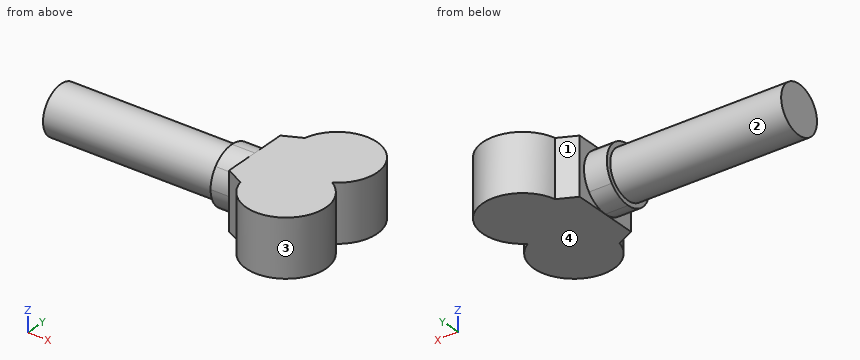
from build123d import *

# Parameters (mm, degrees)
F1_DEPTH = 2.5
F3_DEPTH = 2
F4_R     = 2.1
F5_DEPTH = 15


with BuildPart() as f1:
    # F0 (on Top) → F1 (new body, symmetric)
    with BuildSketch(Plane.XY):
        with BuildLine():
            ThreePointArc((8.1972243623, 3), (10, 2.5), (11.8027756377, 3))
            ThreePointArc((11.8027756377, 3), (10, 3.5), (8.1972243623, 3))
        make_face()
        with BuildLine():
            ThreePointArc((8.1972243623, 3), (6.7824000154, 4.6226654949), (6.584950352, 6.7664436716))
            Line((6.584950352, 6.7664436716), (5, 6))
            Line((5, 6), (5, 3))
            Line((5, 3), (5, 0))
            Line((5, 0), (6.5932639339, -0.8025891701))
            ThreePointArc((6.5932639339, -0.8025891701), (6.7751474224, 1.3602668315), (8.1972243623, 3))
        make_face()
        with BuildLine():
            ThreePointArc((11.8027756377, 3), (13.0462858313, 4.2765898242), (13.5, 6))
            ThreePointArc((13.5, 6), (10.385568562, 9.4786975844), (6.584950352, 6.7664436716))
            ThreePointArc((6.584950352, 6.7664436716), (6.7824000154, 4.6226654949), (8.1972243623, 3))
            ThreePointArc((8.1972243623, 3), (10, 3.5), (11.8027756377, 3))
        make_face()
        with BuildLine():
            ThreePointArc((13.5, 0), (13.0462858313, 1.7234101758), (11.8027756377, 3))
            ThreePointArc((11.8027756377, 3), (10, 2.5), (8.1972243623, 3))
            ThreePointArc((8.1972243623, 3), (6.7751474224, 1.3602668315), (6.5932639339, -0.8025891701))
            ThreePointArc((6.5932639339, -0.8025891701), (10.4039949063, -3.4766058327), (13.5, 0))
        make_face()
    extrude(amount=F1_DEPTH, both=True)

    # F2 (on face) → F3 (join)
    with BuildSketch(Plane(origin=(5, 0, 0), x_dir=(0, -1, 0), z_dir=(-1, 0, 0))):
        with BuildLine():
            ThreePointArc((-0.5, 0), (-0.6493210558, 0.8510631594), (-1.079446801, 1.6004609992))
            Line((-1.079446801, 1.6004609992), (-3, 0))
            Line((-3, 0), (-1.079446801, -1.6004609992))
            ThreePointArc((-1.079446801, -1.6004609992), (-0.6493210558, -0.8510631594), (-0.5, 0))
        make_face()
        with BuildLine():
            Line((-3, 0), (-1.079446801, 1.6004609992))
            ThreePointArc((-1.079446801, 1.6004609992), (-1.9396115094, 2.2639735531), (-3, 2.5))
            ThreePointArc((-3, 2.5), (-4.0603884906, 2.2639735531), (-4.920553199, 1.6004609992))
            Line((-4.920553199, 1.6004609992), (-3, 0))
        make_face()
        with BuildLine():
            Line((-1.079446801, -1.6004609992), (-3, 0))
            Line((-3, 0), (-4.920553199, -1.6004609992))
            ThreePointArc((-4.920553199, -1.6004609992), (-4.0603884906, -2.2639735531), (-3, -2.5))
            ThreePointArc((-3, -2.5), (-1.9396115094, -2.2639735531), (-1.079446801, -1.6004609992))
        make_face()
        with BuildLine():
            Line((-4.920553199, -1.6004609992), (-3, 0))
            Line((-3, 0), (-4.920553199, 1.6004609992))
            ThreePointArc((-4.920553199, 1.6004609992), (-5.5, 0), (-4.920553199, -1.6004609992))
        make_face()
    extrude(amount=F3_DEPTH)

    # F4 (on face) → F5 (join)
    with BuildSketch(Plane(origin=(3, 0, 0), x_dir=(0, -1, 0), z_dir=(-1, 0, 0))):
        with Locations((-3, 0)):
            Circle(F4_R)
    extrude(amount=F5_DEPTH)


solid = f1.part
For this review, take the finished solid that the model builds, in its own axes (mm). Face numbers are marked on the shaded views. Round coordinates to 2 decimals unless told otherwise and drop trailing zeros. Write each loop counter-clockwise with the first axis right and the second up, starting at its lowest first coordinate (ties: lowest second). Pieces come first, ordered by that corner, then holes. Notation, with made-up numbers: M 61.5,-37 L 74.5,-37 A18 ccw 74.5,-15 Z; hole C 54.25,-36 d1. An arc over 180 degrees is marked long. Write item = value, one per line. Start each with the question number.
(1) We need section B-B (z = 1.35). Give the boundary of the cut face in (x, y), then the cut area to 3 significant figures.
(2) The part is to be moulded in two halves that separate along Y. For the marked faces 1, 2, 3 and 4, say which applies: +Y half, -Y half, draft (parallel to the pull), parting line (faces both ways), or undercut.
(3) We need section C-C (y = 1.5). Give the boundary of the cut face in (x, z), then the cut area to 3 significant figures.
(4) Clearance check with flat-ended pins moving along their axes: pin 1 Ø3 at (x, y) = (-5.5, 6) entering from +Z; pin 2 Ø2 at (x, z) = (-3, -1) entering from +Y; pin 3 Ø3 at (x, y) = (-1, 2) entering from -Z. State where each tip first meets the part, or that it passes through.
(5) For line 1 along X through (y, z) = (0.5, 0.9); line 2 along Z through (x, y) = (-4.5, 1.25); line 3 along Y through (x, z) = (7.25, -1.55), list the stretches that pass through material, from the lowest coordinate up.
(6) We need section A-A (x = 4.25). Give the boundary of the cut face in (y, z), then the cut area to 3 significant figures.
(7) We need section D-D (x = -9.5). Give the boundary of the cut face in (y, z), then the cut area to 3 significant figures.
Results found:
q1.outline = M -12,1.39 L 3,1.39 L 3,0.9 L 5,0.9 L 5,0 L 6.59,-0.8 A3.5 ccw long 11.8,3 A3.5 ccw long 6.58,6.77 L 5,6 L 5,5.1 L 3,5.1 L 3,4.61 L -12,4.61 Z
q1.area = 144 mm²
q2.face_1 = +Y half
q2.face_2 = parting line
q2.face_3 = undercut
q2.face_4 = draft
q3.outline = M -12,-1.47 L 3,-1.47 L 3,-2 L 5,-2 L 5,-2.5 L 13.16,-2.5 L 13.16,2.5 L 5,2.5 L 5,2 L 3,2 L 3,1.47 L -12,1.47 Z
q3.area = 92.9 mm²
q4.pin_1 = 1.47
q4.pin_2 = 5.1
q4.pin_3 = -2.1
q5.line_1 = 5 to 13.46
q5.line_2 = -1.16 to 1.16
q5.line_3 = -2.17 to 8.17
q6.outline = C 3,0 d5
q6.area = 19.6 mm²
q7.outline = C 3,0 d4.2
q7.area = 13.9 mm²
